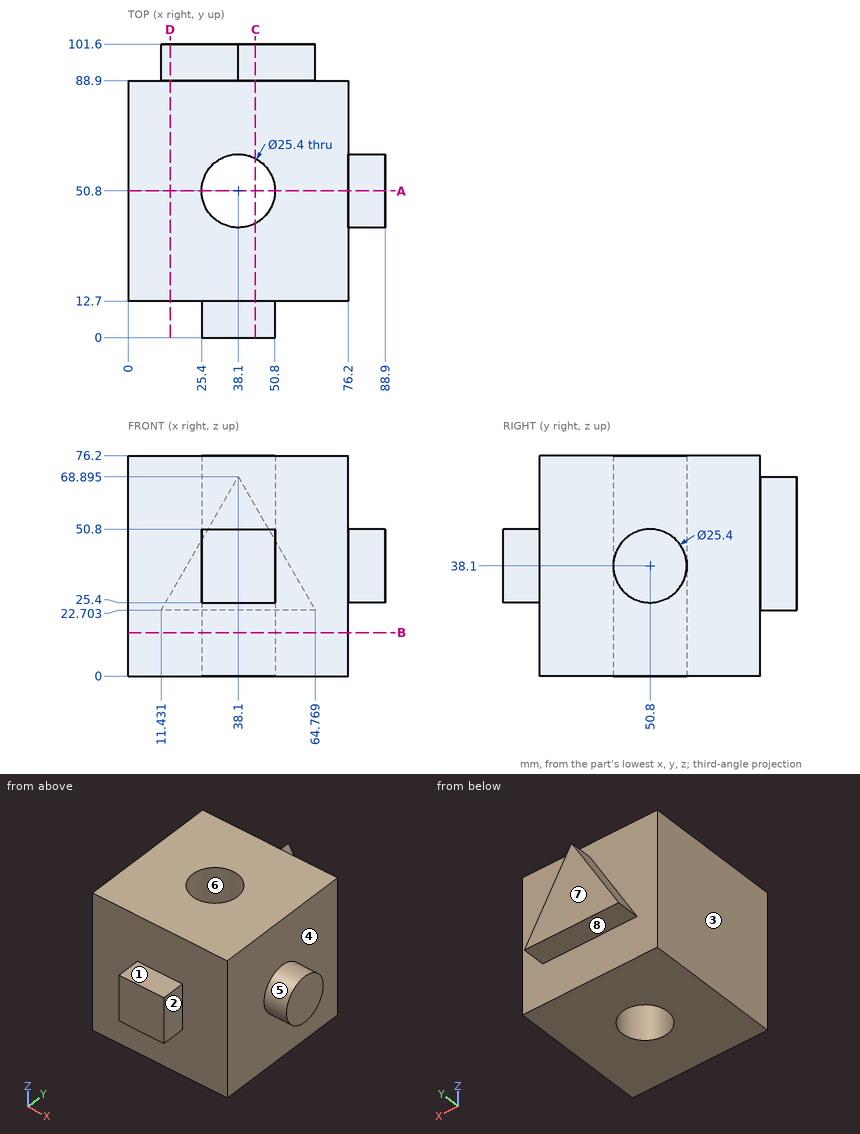
Can you work these out from the drawing? Everything is in mm from the part's minimum corner. A direction names the side the tool comes from. Give positions to 0.01 mm unless a question says otherwise; leave off trailing zeros. Order: outer loops, then holes, each group sorted by start corner. A loop starts at its lowest first (then second) coordinate and runs counter-clockwise, first axis right, second up. Notation, with made-up numbers: (-34.5, 88) -> (7.5, 88) arc R23 cw to (7.5, 105) -> close; hole circle Ø5 at (66.5, 59). An arc over 180 degrees is marked (long way). Return JSON: item names as keys, results as strings.
1. Imagine slicing it at C-C on x = 44. List the corners of the cut face in (y, z) for me (1 decimal).
Answer list:
{"outline": "(0, 25.4) -> (12.7, 25.4) -> (12.7, 0) -> (39.6, 0) -> (39.6, 76.2) -> (12.7, 76.2) -> (12.7, 50.8) -> (0, 50.8) -> close; (62, 0) -> (88.9, 0) -> (88.9, 22.7) -> (101.6, 22.7) -> (101.6, 58.7) -> (88.9, 58.7) -> (88.9, 76.2) -> (62, 76.2) -> close"}
2. Imagine slicing it at B-B on z = 15. List the corners of the cut face in (x, y) for me, then the cut area to 3 significant figures.
Answer list:
{"outline": "(0, 12.7) -> (76.2, 12.7) -> (76.2, 88.9) -> (0, 88.9) -> close; hole circle Ø25.4 at (38.1, 50.8)", "area": "5,300 mm2"}
3. For pin 1 Ø4 at (x, y) = (41, 6.5) entering from -Z; pin 2 Ø10 at (y, z) = (6, 44) entering from +X; pin 3 Ø2 at (y, z) = (42.5, 10.5) entering from +X, each with a flat end and sliding along its axis, tell me the tip position at first contact or that it passes through.
Answer list:
{"pin 1": "stops at z = 25.4", "pin 2": "stops at x = 50.8", "pin 3": "stops at x = 76.2"}
4. I need wall thicknesses on line 1 (Y direction, x = 38, z = 44); line 2 (Y direction, x = 38.1, z = 56.5); line 3 (Y direction, x = 69.5, z = 62.5). Which ranges of each line are inside material? Lowest first, please. Write a range as from..to.
Answer list:
{"line 1": "y = 0..38.1, 63.5..101.6", "line 2": "y = 12.7..38.1, 63.5..101.6", "line 3": "y = 12.7..88.9"}
5. On a 3-axis mill with a long thin cutter (end or side, diameter ignored), from which of +Z, -Z, +X, -X, +Y, -Y can I reach the whole of each face in a straight line? I mean the marked faces 1, 2, 3 and 4. Say none if no direction works.
Answer list:
{"face 1": "+Z, +X, -X, -Y", "face 2": "+Z, -Z, +X, -Y", "face 3": "+Z, -Z, -X, +Y, -Y", "face 4": "+X"}
6. Imagine slicing it at D-D on x = 14.5. List the corners of the cut face in (y, z) for me, then the cut area to 3 significant figures.
Answer list:
{"outline": "(12.7, 0) -> (88.9, 0) -> (88.9, 22.7) -> (101.6, 22.7) -> (101.6, 28.02) -> (88.9, 28.02) -> (88.9, 76.2) -> (12.7, 76.2) -> close", "area": "5,870 mm2"}
7. Imagine slicing it at A-A on y = 50.8. List the corners of the cut face in (x, z) for me, then the cut area to 3 significant figures.
Answer list:
{"outline": "(0, 0) -> (25.4, 0) -> (25.4, 76.2) -> (0, 76.2) -> close; (50.8, 0) -> (76.2, 0) -> (76.2, 25.4) -> (88.9, 25.4) -> (88.9, 50.8) -> (76.2, 50.8) -> (76.2, 76.2) -> (50.8, 76.2) -> close", "area": "4,190 mm2"}
8. Thinking about a two-plate mould opening in Y: for the marked faces 5, 6, 7 and 8, which applies, pulls with the +Y half, pulls with the -Y half, needs draft (parallel to the pull), parting line crosses it, or undercut?
Answer list:
{"face 5": "parting line crosses it", "face 6": "undercut", "face 7": "pulls with the +Y half", "face 8": "needs draft"}
